```python
from build123d import *

# Parameters (mm, degrees)
SKETCH1_R           = 60
BOSS_EXTRUDE1_DEPTH = 5
SKETCH2_R           = 2
SKETCH2_R_2         = 3
CUT_EXTRUDE2_DEPTH  = 5
FILLET1_R           = 7
CUT_EXTRUDE3_DEPTH  = 10


with BuildPart() as part:
    # Sketch1 → Boss-Extrude1 (new body)
    with BuildSketch(Plane.XY):
        Circle(SKETCH1_R)
    extrude(amount=BOSS_EXTRUDE1_DEPTH)

    # Sketch2 → Cut-Extrude2 (cut)
    with BuildSketch(Plane.XY.offset(5)):
        Circle(SKETCH2_R)
        with Locations((0, 50)):
            Circle(SKETCH2_R_2)
        with Locations((15.450849719, 47.552825815)):
            Circle(SKETCH2_R_2)
        with Locations((29.389262615, 40.450849719)):
            Circle(SKETCH2_R_2)
        with Locations((40.450849719, 29.389262615)):
            Circle(SKETCH2_R_2)
        with Locations((47.552825815, 15.450849719)):
            Circle(SKETCH2_R_2)
        with Locations((50, 0)):
            Circle(SKETCH2_R_2)
        with Locations((47.552825815, -15.450849719)):
            Circle(SKETCH2_R_2)
        with Locations((40.450849719, -29.389262615)):
            Circle(SKETCH2_R_2)
        with Locations((29.389262615, -40.450849719)):
            Circle(SKETCH2_R_2)
        with Locations((15.450849719, -47.552825815)):
            Circle(SKETCH2_R_2)
        with Locations((0, -50)):
            Circle(SKETCH2_R_2)
        with Locations((-15.450849719, -47.552825815)):
            Circle(SKETCH2_R_2)
        with Locations((-29.389262615, -40.450849719)):
            Circle(SKETCH2_R_2)
        with Locations((-40.450849719, -29.389262615)):
            Circle(SKETCH2_R_2)
        with Locations((-47.552825815, -15.450849719)):
            Circle(SKETCH2_R_2)
        with Locations((-50, 0)):
            Circle(SKETCH2_R_2)
        with Locations((-47.552825815, 15.450849719)):
            Circle(SKETCH2_R_2)
        with Locations((-40.450849719, 29.389262615)):
            Circle(SKETCH2_R_2)
        with Locations((-29.389262615, 40.450849719)):
            Circle(SKETCH2_R_2)
        with Locations((-15.450849719, 47.552825815)):
            Circle(SKETCH2_R_2)
        with BuildLine():
            Line((-26.704527531, 32.073997698), (-6.627939737, 11.997409903))
            ThreePointArc((-6.627939737, 11.997409903), (-9.691940712, 9.691940712), (-11.997409903, 6.627939737))
            Line((-11.997409903, 6.627939737), (-32.073997698, 26.704527531))
            ThreePointArc((-32.073997698, 26.704527531), (-32.073997698, 32.073997698), (-26.704527531, 32.073997698))
        make_face()
        with BuildLine():
            Line((3.796788766, 41.562693778), (3.796788766, 13.170111032))
            ThreePointArc((3.796788766, 13.170111032), (0, 13.706474001), (-3.796788766, 13.170111032))
            Line((-3.796788766, 13.170111032), (-3.796788766, 41.562693778))
            ThreePointArc((-3.796788766, 41.562693778), (0, 45.359482544), (3.796788766, 41.562693778))
        make_face()
        with BuildLine():
            Line((32.073997698, 26.704527531), (11.997409903, 6.627939737))
            ThreePointArc((11.997409903, 6.627939737), (9.691940712, 9.691940712), (6.627939737, 11.997409903))
            Line((6.627939737, 11.997409903), (26.704527531, 32.073997698))
            ThreePointArc((26.704527531, 32.073997698), (32.073997698, 32.073997698), (32.073997698, 26.704527531))
        make_face()
        with BuildLine():
            Line((41.562693778, -3.796788766), (13.170111032, -3.796788766))
            ThreePointArc((13.170111032, -3.796788766), (13.706474001, 0), (13.170111032, 3.796788766))
            Line((13.170111032, 3.796788766), (41.562693778, 3.796788766))
            ThreePointArc((41.562693778, 3.796788766), (45.359482544, 0), (41.562693778, -3.796788766))
        make_face()
        with BuildLine():
            Line((26.704527531, -32.073997698), (6.627939737, -11.997409903))
            ThreePointArc((6.627939737, -11.997409903), (9.691940712, -9.691940712), (11.997409903, -6.627939737))
            Line((11.997409903, -6.627939737), (32.073997698, -26.704527531))
            ThreePointArc((32.073997698, -26.704527531), (32.073997698, -32.073997698), (26.704527531, -32.073997698))
        make_face()
        with BuildLine():
            Line((-3.796788766, -41.562693778), (-3.796788766, -13.170111032))
            ThreePointArc((-3.796788766, -13.170111032), (0, -13.706474001), (3.796788766, -13.170111032))
            Line((3.796788766, -13.170111032), (3.796788766, -41.562693778))
            ThreePointArc((3.796788766, -41.562693778), (0, -45.359482544), (-3.796788766, -41.562693778))
        make_face()
        with BuildLine():
            Line((-32.073997698, -26.704527531), (-11.997409903, -6.627939737))
            ThreePointArc((-11.997409903, -6.627939737), (-9.691940712, -9.691940712), (-6.627939737, -11.997409903))
            Line((-6.627939737, -11.997409903), (-26.704527531, -32.073997698))
            ThreePointArc((-26.704527531, -32.073997698), (-32.073997698, -32.073997698), (-32.073997698, -26.704527531))
        make_face()
        with BuildLine():
            Line((-41.562693778, 3.796788766), (-13.170111032, 3.796788766))
            ThreePointArc((-13.170111032, 3.796788766), (-13.706474001, 0), (-13.170111032, -3.796788766))
            Line((-13.170111032, -3.796788766), (-41.562693778, -3.796788766))
            ThreePointArc((-41.562693778, -3.796788766), (-45.359482544, 0), (-41.562693778, 3.796788766))
        make_face()
    extrude(amount=-CUT_EXTRUDE2_DEPTH, mode=Mode.SUBTRACT)

    # Fillet1
    # the kernel refuses this fillet: 7 mm, written as the material it adds along each edge
    with BuildSketch(Plane(origin=(11.997409903, 6.627939737, 5), x_dir=(-0.6614265480473352, 0.7500099476261538, 0), z_dir=(0, 0, -1)), Plane(origin=(13.170111032, -3.796788766, 5), x_dir=(0.06263792254265388, 0.9980363173049068, 0), z_dir=(0, 0, -1)), Plane(origin=(6.627939737, -11.997409903, 5), x_dir=(0.7500099476260863, 0.661426548047412, 0), z_dir=(0, 0, -1)), Plane(origin=(-3.796788766, -13.170111032, 5), x_dir=(0.998036317304904, -0.06263792254269633, 0), z_dir=(0, 0, -1)), Plane(origin=(-11.997409903, -6.627939737, 5), x_dir=(0.6614265480472753, -0.7500099476262067, 0), z_dir=(0, 0, -1)), Plane(origin=(-13.170111032, 3.796788766, 5), x_dir=(-0.06263792254277421, -0.9980363173048992, 0), z_dir=(0, 0, -1)), Plane(origin=(-6.627939737, 11.997409903, 5), x_dir=(-0.7500099476261984, -0.6614265480472847, 0), z_dir=(0, 0, -1)), Plane(origin=(3.796788766, 13.170111032, 5), x_dir=(-0.9980363173048974, 0.06263792254280169, 0), z_dir=(0, 0, -1))) as fillet1_piece_1:
        with BuildLine():
            CenterArc((7.442703057, 6.834325481), FILLET1_R, 176.408760408, 81.100827227)
            Line((0.456448836, 7.272790939), (0, 0))
            ThreePointArc((0, 0), (2.964384683, 0.324401927), (5.928769366, 0))
        make_face()
    extrude(amount=5)
    with BuildSketch(Plane(origin=(6.627939737, 11.997409903, 5), x_dir=(0.7071067811865476, 0.7071067811865476, 0), z_dir=(0, 0, -1)), Plane(origin=(13.170111032, 3.796788766, 5), x_dir=(1, 0, 0), z_dir=(0, 0, -1)), Plane(origin=(-6.627939737, -11.997409903, 5), x_dir=(-0.7071067811865477, -0.7071067811865474, 0), z_dir=(0, 0, -1)), Plane(origin=(-13.170111032, -3.796788766, 5), x_dir=(-1, 0, 0), z_dir=(0, 0, -1)), Plane(origin=(-3.796788766, 13.170111032, 5), x_dir=(0, 1, 0), z_dir=(0, 0, -1))) as fillet1_piece_2:
        with BuildLine():
            CenterArc((7.287100492, 7), FILLET1_R, 188.899172773, 81.100827227)
            ThreePointArc((0.371365796, 5.917127144), (0.509447803, 2.938243709), (0, 0))
            Line((0, 0), (7.287100492, 0))
        make_face()
    extrude(amount=5)
    with BuildSketch(Plane(origin=(11.997409903, -6.627939737, 5), x_dir=(-0.661426548047024, -0.7500099476264284, 0), z_dir=(0, 0, -1)), Plane(origin=(3.796788766, -13.170111032, 5), x_dir=(-0.9980363173048815, -0.06263792254305393, 0), z_dir=(0, 0, -1)), Plane(origin=(-11.997409903, 6.627939737, 5), x_dir=(0.6614265480472289, 0.7500099476262477, 0), z_dir=(0, 0, -1))) as fillet1_piece_3:
        with BuildLine():
            CenterArc((7.442703057, -6.834325481), FILLET1_R, 102.490412365, 81.100827227)
            Line((0.456448836, -7.272790939), (0, 0))
            ThreePointArc((0, 0), (2.964384683, -0.324401927), (5.928769366, 0))
        make_face()
    extrude(amount=5)

    # Sketch3 → Cut-Extrude3 (cut)
    with BuildSketch(Plane.XY.offset(5)):
        Polygon((0, 6.92820323), (-6, 3.464101615), (-6, -3.464101615), (0, -6.92820323), (6, -3.464101615), (6, 3.464101615), align=None)
    extrude(amount=-CUT_EXTRUDE3_DEPTH, mode=Mode.SUBTRACT)


solid = part.part
```
Here's how the part is built. I have some questions about the finished solid (model axes, mm). Coordinates: 2 decimals unless noted, no trailing zeros. Order: outer loops, then holes, each group sorted by start corner. A loop starts at its lowest first (then second) coordinate and runs counter-clockwise, first axis right, second up.
1) Will these pins go through, and if not, where does the flat tip stop? pin 1 (5 mm diameter, centred on x = -50, y = 0, fed in from -Z); pin 2 (2.5 mm diameter, centred on x = 30.5, z = 2, fed in from -Y); pin 3 (1.5 mm diameter, centred on y = -26.5, z = 1.5, fed in from -X); pin 4 (1.5 mm diameter, centred on x = -22, z = 3.5, fed in from -Y).
2) Imagine slicing it at B-B on z = 2.6. State how many separate pieces and enclosed holes the cut face has, and give its area (3 significant figures).
3) I need wall thicknesses on line 1 (X direction, y = -2, z = 0.65); line 2 (Y direction, x = -13, z = 4); line 3 (Y direction, x = 22.5, z = 0.45). Which ranges of each line are inside material? Lowest first, please.
4) Imagine slicing it at A-A on x = -29.5. List the corners of the cut face in (y, z) for me.
5) We'd pull the mould along Y, two halves only. Please class faces 1 (the face through (9, -9, 5)), 2 (the face through (2.745, -16.766, 2.535)): +Y half, -Y half, draft (parallel to the pull), parting line (faces both ways), or undercut.
Response values:
1. pin 1: passes through
1. pin 2: stops at y = -52.39
1. pin 3: stops at x = -54.19
1. pin 4: stops at y = -56.11
2. separate pieces: 1
2. enclosed holes: 29
2. area: 8,890 mm2
3. line 1: x = -59.97 to -52.24, -47.76 to -44.79, -15.77 to -6, 6 to 15.77, 44.79 to 47.76, 52.24 to 59.97
3. line 2: y = -58.57 to -49.28, -45.82 to -18.37, -9.78 to 9.78, 18.37 to 45.82, 49.28 to 58.57
3. line 3: y = -55.62 to -27.87, -17.13 to -3.8, 3.8 to 17.13, 27.87 to 55.62
4. outline: (-52.25, 0) - (-43.45, 0) - (-43.45, 5) - (-52.25, 5) - close; (-37.45, 0) - (-33.18, 0) - (-33.18, 5) - (-37.45, 5) - close; (-24.13, 0) - (-3.8, 0) - (-3.8, 5) - (-24.13, 5) - close; (3.8, 0) - (24.13, 0) - (24.13, 5) - (3.8, 5) - close; (33.18, 0) - (37.45, 0) - (37.45, 5) - (33.18, 5) - close; (43.45, 0) - (52.25, 0) - (52.25, 5) - (43.45, 5) - close
5. face 1: draft
5. face 2: undercut
